from build123d import *

# Parameters (mm, degrees)
F0_W     = 80
F0_H     = 180
F1_DEPTH = 15
F2_R     = 3
F3_DEPTH = 15.001
F4_R     = 3
F5_DEPTH = 80.001


with BuildPart() as f1:
    # F0 (on Front) → F1 (new body)
    with BuildSketch(Plane.XZ):
        with Locations((40, 90)):
            Rectangle(F0_W, F0_H)
    extrude(amount=F1_DEPTH)

    # F2 (on face) → F3 (cut, through all)
    with BuildSketch(Plane.XZ.offset(15)):
        with Locations((60, 6)):
            Circle(F2_R)
        with Locations((20, 6)):
            Circle(F2_R)
    extrude(amount=-F3_DEPTH, mode=Mode.SUBTRACT)

    # F4 (on face) → F5 (cut, through all)
    with BuildSketch(Plane(origin=(0, 0, 0), x_dir=(0, -1, 0), z_dir=(-1, 0, 0))):
        with Locations((7.5, 30)):
            Circle(F4_R)
        with Locations((7.5, 150)):
            Circle(F4_R)
    extrude(amount=-F5_DEPTH, mode=Mode.SUBTRACT)


solid = f1.part
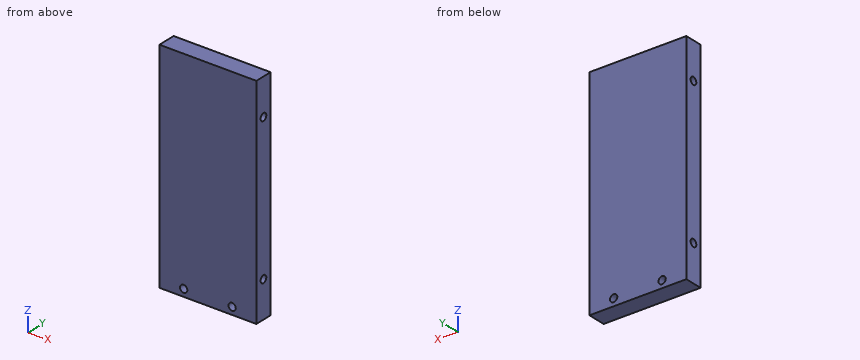
Work out the finished part from the listing and answer in its coordinate system (mm). Round coordinates to 2 decimals unless told otherwise and drop trailing zeros. Write each loop counter-clockwise with the first axis right and the second up, starting at its lowest first coordinate (ties: lowest second). Pieces come first, ordered by that corner, then holes. Notation, with made-up numbers: (74.5, -29) -> (119.5, -29) arc R22 ccw to (119.5, -5) -> close; hole circle Ø6 at (44.25, -4). An arc over 180 degrees is marked (long way). Answer as CSV lines item,"result". Start each with the question number.
(1) The part is cut by section B-B, the plane y = -7.5. Give the vertices of the cut face in (x, z), then the cut area to 3 significant figures.
(2) Find the intervals of material crossed by probe 1 along Z at (x, y) = (34.5, -7.5); probe 2 along Y at (x, z) = (48, 150); probe 3 along Z at (x, y) = (60, -10.25), in increasing order.
(3) The part is cut by section A-A, the plane x = 20. Give the vertices of the cut face in (y, z).
(4) This flat-tipped pin is pushed along its axis until it touches: pin 1 (5.5 mm diameter, centred on x = 60, z = 6, fed in from +Y). Where does it stop, or does it pass through?
(5) The part is cut by section D-D, the plane z = 150. Give the vertices of the cut face in (x, y).
(6) The part is cut by section C-C, the plane z = 6. Give the vertices of the cut face in (x, y), then the cut area to 3 significant figures.
Output values:
1,outline,"(0, 0) -> (80, 0) -> (80, 27) -> (0, 27) -> close; (0, 33) -> (80, 33) -> (80, 147) -> (0, 147) -> close; (0, 153) -> (80, 153) -> (80, 180) -> (0, 180) -> close; hole circle Ø6 at (20, 6); hole circle Ø6 at (60, 6)"
1,area,"13,400 mm²"
2,probe 1,"z = 0 to 27, 33 to 147, 153 to 180"
2,probe 2,"y = -15 to -10.5, -4.5 to 0"
2,probe 3,"z = 0 to 3, 9 to 28.8, 31.2 to 148.8, 151.2 to 180"
3,outline,"(-15, 0) -> (0, 0) -> (0, 3) -> (-15, 3) -> close; (-15, 9) -> (0, 9) -> (0, 180) -> (-15, 180) -> close; hole circle Ø6 at (-7.5, 30); hole circle Ø6 at (-7.5, 150)"
4,pin 1,"passes through"
5,outline,"(0, -15) -> (80, -15) -> (80, -10.5) -> (0, -10.5) -> close; (0, -4.5) -> (80, -4.5) -> (80, 0) -> (0, 0) -> close"
6,outline,"(0, -15) -> (17, -15) -> (17, 0) -> (0, 0) -> close; (23, -15) -> (57, -15) -> (57, 0) -> (23, 0) -> close; (63, -15) -> (80, -15) -> (80, 0) -> (63, 0) -> close"
6,area,"1,020 mm²"
